Source: three-view drawing plus pictorial views. Frame: mm from the lowest corner of the part. A direction names the side the tool comes from. Coordinates: 2 decimals unless noted, no trailing zeros. Order: outer loops, then holes, each group sorted by start corner. A loop starts at its lowest first (then second) coordinate and runs counter-clockwise, first axis right, second up. Notation, with made-up numbers: (23, 43.5) -> (81, 43.5) arc R22 cw to (81, 78.5) -> close; hole circle Ø8 at (25, -3). An arc over 180 degrees is marked (long way). Use CSV: the item, a comma, the result in double quotes. Start each with the question number.
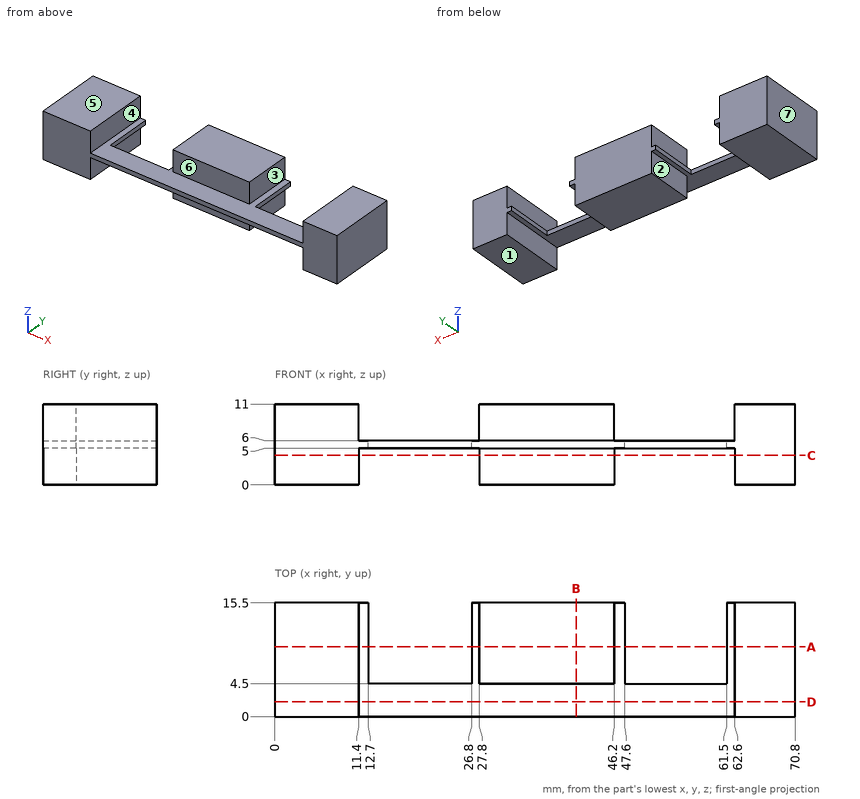
1. Section C-C on z = 4. Return loops of the section in (x, y).
2. Access query for the marked faces 1, 2 and 3. Directions: +Z, -Z, +X, -X, +Y, -Y. A direction counts if a zero-diameter tool reaches every point of the face in a straight line with its end or side. Return the directions, or none.
3. Material intervals for line 1 along X through (y, z) = (14, 9); line 2 along X through (y, z) = (1.75, 2.5); line 3 along Z through (x, y) = (12.5, 6.5), sorted ascending.
4. Contact query for flat-ended pins moving along their axis: P1, Ø1.5, axis at x = 38, z = 9.5, coming from the -Y side; P2, Ø0.5, axis at x = 51, z = 5.5, coming from the +Y side; P3, Ø1.5, axis at x = 30, y = 3, coming from the +Z side. Output: stop coordinate, or through.
5. Section D-D on y = 2. Return loops of the section in (x, z), then the cut area to 3 significant figures.
6. Section B-B on x = 41. Return loops of the section in (y, z), then the cut area to 4 significant figures.
7. Section A-A on y = 9.5. Return loops of the section in (x, z), then the cut area to 3 significant figures.
8. Pull-direction query (X, two-part tool) for the marked faces 4, 5, 6 and 7; classes: released by +X, released by -X, zero draft, split by the parting line, or undercut.
Values follow:
1,outline,"(0, 0) -> (11.4, 0) -> (11.4, 15.5) -> (0, 15.5) -> close; (27.8, 4.5) -> (46.2, 4.5) -> (46.2, 15.5) -> (27.8, 15.5) -> close; (62.6, 0) -> (70.8, 0) -> (70.8, 15.5) -> (62.6, 15.5) -> close"
2,face 1,"-Z, +X, -X, +Y, -Y"
2,face 2,"-Z, +Y, -Y"
2,face 3,"+Z, +Y, -Y"
3,line 1,"x = 0 to 11.4, 27.8 to 46.2, 62.6 to 70.8"
3,line 2,"x = 0 to 11.4, 62.6 to 70.8"
3,line 3,"z = 5 to 6"
4,P1,"stops at y = 4.5"
4,P2,"stops at y = 4.5"
4,P3,"stops at z = 6"
5,outline,"(0, 0) -> (11.4, 0) -> (11.4, 5) -> (62.6, 5) -> (62.6, 0) -> (70.8, 0) -> (70.8, 11) -> (62.6, 11) -> (62.6, 6) -> (11.4, 6) -> (11.4, 11) -> (0, 11) -> close"
5,area,"267 mm2"
6,outline,"(0, 5) -> (4.5, 5) -> (4.5, 0) -> (15.5, 0) -> (15.5, 11) -> (4.5, 11) -> (4.5, 6) -> (0, 6) -> close"
6,area,"125.5 mm2"
7,outline,"(0, 0) -> (11.4, 0) -> (11.4, 5) -> (12.7, 5) -> (12.7, 6) -> (11.4, 6) -> (11.4, 11) -> (0, 11) -> close; (26.8, 5) -> (27.8, 5) -> (27.8, 0) -> (46.2, 0) -> (46.2, 5) -> (47.6, 5) -> (47.6, 6) -> (46.2, 6) -> (46.2, 11) -> (27.8, 11) -> (27.8, 6) -> (26.8, 6) -> close; (61.5, 5) -> (62.6, 5) -> (62.6, 0) -> (70.8, 0) -> (70.8, 11) -> (62.6, 11) -> (62.6, 6) -> (61.5, 6) -> close"
7,area,"423 mm2"
8,face 4,"undercut"
8,face 5,"zero draft"
8,face 6,"undercut"
8,face 7,"released by -X"
